Read the model definition and answer for the solid it produces. Units are mm, in the model's axes. Give positions to 0.01 mm unless a question says otherwise; leave off trailing zeros. Order: outer loops, then holes, each group sorted by start corner. A loop starts at its lowest first (then second) coordinate and runs counter-clockwise, first axis right, second up.
Item 1: Find the intervals of material crossed by line 1 along Y through (x, z) = (22.5, 8); line 2 along Y through (x, z) = (120, 7.5); line 3 along X through (y, z) = (3, 6.5), in increasing order.
Item 2: Given pin 1 Ø5.5 at (x, y) = (44.45, 139.7) entering from -Z; pin 2 Ø4 at (y, z) = (0.5, 10.5) entering from -X, each flat-ended and moving along its own axis, determine where each tip first touches the part or whether it passes through.
Item 3: A cutting plane is placed at C-C (x = 120.65). Write down the section's boundary in (y, z) (3 decimals).
Item 4: A cutting plane is placed at A-A (x = 44.45). Write down the section's boundary in (y, z) (3 decimals).
Item 5: A cutting plane is placed at D-D (z = 3). State how many separate pieces and enclosed holes the cut face has, plus the area to 3 significant figures.
Item 6: A cutting plane is placed at B-B (y = 12.7). Write down the section's boundary in (x, z) (3 decimals), plus the area to 3 significant figures.
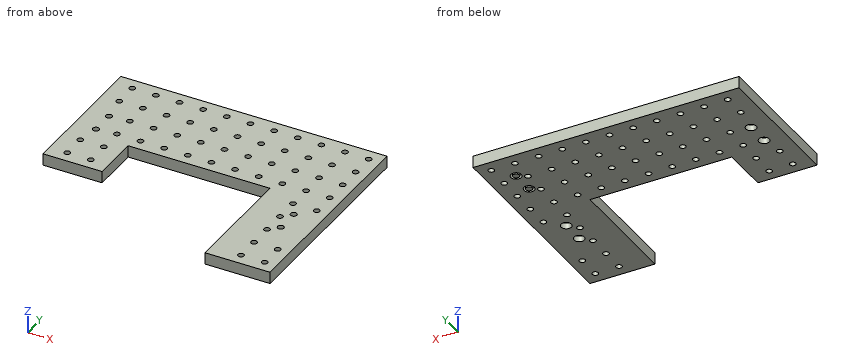
from build123d import *

# Parameters (mm, degrees)
SKETCH1_R           = 3.175
BOSS_EXTRUDE1_DEPTH = 12.7
SKETCH2_R           = 3.175
CUT_EXTRUDE1_DEPTH  = 12.7
SKETCH3_R           = 3.3734375
CUT_EXTRUDE2_DEPTH  = 12.7
CUT_EXTRUDE3_START  = -6.35
SKETCH3_3_R         = 5.55625
SKETCH3_3_R_2       = 3.3734375
SKETCH3_3_R_3       = 5.588
SKETCH3_3_R_4       = 3.429
CUT_EXTRUDE3_DEPTH  = 6.35
SKETCH5_R           = 3.3734375
CUT_EXTRUDE4_DEPTH  = 12.7
SKETCH5_3_R         = 5.55625
SKETCH5_3_R_2       = 3.3734375
CUT_EXTRUDE5_DEPTH  = 6.35


with BuildPart() as part:
    # Sketch1 → Boss-Extrude1 (new body)
    with BuildSketch(Plane.XY):
        Polygon((0, 152.4), (0, 0), (63.5, 0), (63.5, 50.8), (215.9, 50.8), (215.9, -76.2), (285.75, -76.2), (285.75, 152.4), align=None)
        with Locations((19.05, 12.7)):
            Circle(SKETCH1_R, mode=Mode.SUBTRACT)
        with Locations((19.05, 38.1)):
            Circle(SKETCH1_R, mode=Mode.SUBTRACT)
        with Locations((44.45, 12.7)):
            Circle(SKETCH1_R, mode=Mode.SUBTRACT)
        with Locations((44.45, 38.1)):
            Circle(SKETCH1_R, mode=Mode.SUBTRACT)
        with Locations((247.65, 12.7)):
            Circle(SKETCH1_R, mode=Mode.SUBTRACT)
        with Locations((247.65, 38.1)):
            Circle(SKETCH1_R, mode=Mode.SUBTRACT)
        with Locations((44.45, 63.5)):
            Circle(SKETCH1_R, mode=Mode.SUBTRACT)
        with Locations((69.85, 63.5)):
            Circle(SKETCH1_R, mode=Mode.SUBTRACT)
        with Locations((44.45, 88.9)):
            Circle(SKETCH1_R, mode=Mode.SUBTRACT)
        with Locations((69.85, 88.9)):
            Circle(SKETCH1_R, mode=Mode.SUBTRACT)
        with Locations((95.25, 63.5)):
            Circle(SKETCH1_R, mode=Mode.SUBTRACT)
        with Locations((120.65, 63.5)):
            Circle(SKETCH1_R, mode=Mode.SUBTRACT)
        with Locations((95.25, 88.9)):
            Circle(SKETCH1_R, mode=Mode.SUBTRACT)
        with Locations((120.65, 88.9)):
            Circle(SKETCH1_R, mode=Mode.SUBTRACT)
        with Locations((19.05, 114.3)):
            Circle(SKETCH1_R, mode=Mode.SUBTRACT)
        with Locations((44.45, 114.3)):
            Circle(SKETCH1_R, mode=Mode.SUBTRACT)
        with Locations((69.85, 114.3)):
            Circle(SKETCH1_R, mode=Mode.SUBTRACT)
        with Locations((19.05, 139.7)):
            Circle(SKETCH1_R, mode=Mode.SUBTRACT)
        with Locations((44.45, 139.7)):
            Circle(SKETCH1_R, mode=Mode.SUBTRACT)
        with Locations((69.85, 139.7)):
            Circle(SKETCH1_R, mode=Mode.SUBTRACT)
        with Locations((95.25, 114.3)):
            Circle(SKETCH1_R, mode=Mode.SUBTRACT)
        with Locations((120.65, 114.3)):
            Circle(SKETCH1_R, mode=Mode.SUBTRACT)
        with Locations((95.25, 139.7)):
            Circle(SKETCH1_R, mode=Mode.SUBTRACT)
        with Locations((120.65, 139.7)):
            Circle(SKETCH1_R, mode=Mode.SUBTRACT)
        with Locations((146.05, 63.5)):
            Circle(SKETCH1_R, mode=Mode.SUBTRACT)
        with Locations((171.45, 63.5)):
            Circle(SKETCH1_R, mode=Mode.SUBTRACT)
        with Locations((196.85, 63.5)):
            Circle(SKETCH1_R, mode=Mode.SUBTRACT)
        with Locations((146.05, 88.9)):
            Circle(SKETCH1_R, mode=Mode.SUBTRACT)
        with Locations((171.45, 88.9)):
            Circle(SKETCH1_R, mode=Mode.SUBTRACT)
        with Locations((196.85, 88.9)):
            Circle(SKETCH1_R, mode=Mode.SUBTRACT)
        with Locations((222.25, 63.5)):
            Circle(SKETCH1_R, mode=Mode.SUBTRACT)
        with Locations((247.65, 63.5)):
            Circle(SKETCH1_R, mode=Mode.SUBTRACT)
        with Locations((273.05, 63.5)):
            Circle(SKETCH1_R, mode=Mode.SUBTRACT)
        with Locations((222.25, 88.9)):
            Circle(SKETCH1_R, mode=Mode.SUBTRACT)
        with Locations((247.65, 88.9)):
            Circle(SKETCH1_R, mode=Mode.SUBTRACT)
        with Locations((273.05, 88.9)):
            Circle(SKETCH1_R, mode=Mode.SUBTRACT)
        with Locations((146.05, 114.3)):
            Circle(SKETCH1_R, mode=Mode.SUBTRACT)
        with Locations((171.45, 114.3)):
            Circle(SKETCH1_R, mode=Mode.SUBTRACT)
        with Locations((196.85, 114.3)):
            Circle(SKETCH1_R, mode=Mode.SUBTRACT)
        with Locations((146.05, 139.7)):
            Circle(SKETCH1_R, mode=Mode.SUBTRACT)
        with Locations((171.45, 139.7)):
            Circle(SKETCH1_R, mode=Mode.SUBTRACT)
        with Locations((196.85, 139.7)):
            Circle(SKETCH1_R, mode=Mode.SUBTRACT)
        with Locations((222.25, 114.3)):
            Circle(SKETCH1_R, mode=Mode.SUBTRACT)
        with Locations((247.65, 114.3)):
            Circle(SKETCH1_R, mode=Mode.SUBTRACT)
        with Locations((273.05, 114.3)):
            Circle(SKETCH1_R, mode=Mode.SUBTRACT)
        with Locations((222.25, 139.7)):
            Circle(SKETCH1_R, mode=Mode.SUBTRACT)
        with Locations((247.65, 139.7)):
            Circle(SKETCH1_R, mode=Mode.SUBTRACT)
        with Locations((273.05, 139.7)):
            Circle(SKETCH1_R, mode=Mode.SUBTRACT)
    extrude(amount=BOSS_EXTRUDE1_DEPTH)

    # Sketch2 → Cut-Extrude1 (cut)
    with BuildSketch(Plane.XY.offset(12.7)):
        with Locations((247.65, -12.7)):
            Circle(SKETCH2_R)
        with Locations((247.65, -38.1)):
            Circle(SKETCH2_R)
        with Locations((247.65, -63.5)):
            Circle(SKETCH2_R)
        with Locations((273.05, -38.1)):
            Circle(SKETCH2_R)
        with Locations((273.05, -63.5)):
            Circle(SKETCH2_R)
        with Locations((273.05, 38.1)):
            Circle(SKETCH2_R)
    extrude(amount=-CUT_EXTRUDE1_DEPTH, mode=Mode.SUBTRACT)

    # Sketch3 → Cut-Extrude2 (cut)
    with BuildSketch(Plane.XY.offset(12.7)):
        with Locations((257.175, -3.2258)):
            Circle(SKETCH3_R)
        with Locations((257.175, 22.1742)):
            Circle(SKETCH3_R)
    extrude(amount=-CUT_EXTRUDE2_DEPTH, mode=Mode.SUBTRACT)

    # Sketch3<3> → Cut-Extrude3 (cut)
    # profile 1 of 4: a face of its own
    with BuildSketch(Plane.XY.offset(12.7).offset(CUT_EXTRUDE3_START)):
        with Locations((257.175, -3.2258)):
            Circle(SKETCH3_3_R)
        with Locations((257.175, -3.2258)):
            Circle(SKETCH3_3_R_2, mode=Mode.SUBTRACT)
    # profile 2 of 4: a face of its own
    with BuildSketch(Plane.XY.offset(12.7).offset(CUT_EXTRUDE3_START)):
        with Locations((257.175, 22.1742)):
            Circle(SKETCH3_3_R)
        with Locations((257.175, 22.1742)):
            Circle(SKETCH3_3_R_2, mode=Mode.SUBTRACT)
    # profile 3 of 4: a face of its own
    with BuildSketch(Plane.XY.offset(12.7).offset(CUT_EXTRUDE3_START)):
        with Locations((257.175, 120.082847609)):
            Circle(SKETCH3_3_R_3)
        with Locations((257.175, 120.082847609)):
            Circle(SKETCH3_3_R_4, mode=Mode.SUBTRACT)
    # profile 4 of 4: a face of its own
    with BuildSketch(Plane.XY.offset(12.7).offset(CUT_EXTRUDE3_START)):
        with Locations((257.175, 94.682847609)):
            Circle(SKETCH3_3_R_3)
        with Locations((257.175, 94.682847609)):
            Circle(SKETCH3_3_R_4, mode=Mode.SUBTRACT)
    extrude(amount=-CUT_EXTRUDE3_DEPTH, mode=Mode.SUBTRACT)

    # Sketch5 → Cut-Extrude4 (cut)
    with BuildSketch(Plane(origin=(0, 0, 0), x_dir=(-1, 0, 0), z_dir=(0, 0, -1))):
        with Locations((-23.114, 61.3918)):
            Circle(SKETCH5_R)
        with Locations((-23.114, 86.7918)):
            Circle(SKETCH5_R)
    extrude(amount=-CUT_EXTRUDE4_DEPTH, mode=Mode.SUBTRACT)

    # Sketch5<3> → Cut-Extrude5 (cut)
    # profile 1 of 2: a face of its own
    with BuildSketch(Plane(origin=(0, 0, 0), x_dir=(-1, 0, 0), z_dir=(0, 0, -1))):
        with Locations(Location((-23.114, 61.3918, 0), (0, 0, 180))):
            Circle(SKETCH5_3_R)
        with Locations((-23.114, 61.3918)):
            Circle(SKETCH5_3_R_2, mode=Mode.SUBTRACT)
    # profile 2 of 2: a face of its own
    with BuildSketch(Plane(origin=(0, 0, 0), x_dir=(-1, 0, 0), z_dir=(0, 0, -1))):
        with Locations(Location((-23.114, 86.7918, 0), (0, 0, 180))):
            Circle(SKETCH5_3_R)
        with Locations((-23.114, 86.7918)):
            Circle(SKETCH5_3_R_2, mode=Mode.SUBTRACT)
    extrude(amount=-CUT_EXTRUDE5_DEPTH, mode=Mode.SUBTRACT)


solid = part.part
Response values:
1. line 1: y = 0 to 58.07, 64.71 to 83.47, 90.11 to 152.4
1. line 2: y = 50.8 to 60.39, 66.61 to 85.79, 92.01 to 111.19, 117.41 to 136.59, 142.81 to 152.4
1. line 3: x = 0 to 63.5, 215.9 to 285.75
2. pin 1: passes through
2. pin 2: stops at x = 0
3. outline: (50.8, 0) - (60.325, 0) - (60.325, 12.7) - (50.8, 12.7) - close; (66.675, 0) - (85.725, 0) - (85.725, 12.7) - (66.675, 12.7) - close; (92.075, 0) - (111.125, 0) - (111.125, 12.7) - (92.075, 12.7) - close; (117.475, 0) - (136.525, 0) - (136.525, 12.7) - (117.475, 12.7) - close; (142.875, 0) - (152.4, 0) - (152.4, 12.7) - (142.875, 12.7) - close
4. outline: (0, 0) - (9.525, 0) - (9.525, 12.7) - (0, 12.7) - close; (15.875, 0) - (34.925, 0) - (34.925, 12.7) - (15.875, 12.7) - close; (41.275, 0) - (60.325, 0) - (60.325, 12.7) - (41.275, 12.7) - close; (66.675, 0) - (85.725, 0) - (85.725, 12.7) - (66.675, 12.7) - close; (92.075, 0) - (111.125, 0) - (111.125, 12.7) - (92.075, 12.7) - close; (117.475, 0) - (136.525, 0) - (136.525, 12.7) - (117.475, 12.7) - close; (142.875, 0) - (152.4, 0) - (152.4, 12.7) - (142.875, 12.7) - close
5. separate pieces: 3
5. enclosed holes: 60
5. area: 38,900 mm2
6. outline: (0, 0) - (15.875, 0) - (15.875, 12.7) - (0, 12.7) - close; (22.225, 0) - (41.275, 0) - (41.275, 12.7) - (22.225, 12.7) - close; (47.625, 0) - (63.5, 0) - (63.5, 12.7) - (47.625, 12.7) - close; (215.9, 0) - (244.475, 0) - (244.475, 12.7) - (215.9, 12.7) - close; (250.825, 0) - (285.75, 0) - (285.75, 12.7) - (250.825, 12.7) - close
6. area: 1,450 mm2
